Read the model definition and answer for the solid it produces. Units are mm, in the model's axes. Face numbers are marked on the shaded views. A direction names the side the tool comes from. Round coordinates to 2 decimals unless told otherwise and drop trailing zeros. Loops run counter-clockwise (first coordinate to the right, second up) from the corner with the lowest first, then second, coordinate; pieces in that order, holes last. Notation, with made-up numbers: (37, 24.25) - (75, 24.25) arc R30 cw to (75, 62.25) - close; hole circle Ø10 at (-32.5, 69). An arc over 180 degrees is marked (long way). Use one line per item in the form item = value. Start each with the question number.
```python
from build123d import *

# Parameters (mm, degrees)
SKETCH_W          = 46
SKETCH_H          = 22
PAD_DEPTH         = 20
SKETCH001_W       = 41
SKETCH001_H       = 17
POCKET_DEPTH      = 0.001
POCKET_DEPTH_BACK = 20.001
SKETCH002_R       = 3.62
POCKET001_DEPTH   = 3.5
SKETCH003_R       = 2
POCKET002_DEPTH   = 2.5
CHAMFER_SIZE      = 2.485
FILLET_R          = 1


with BuildPart() as part:
    # Sketch → Pad (new body)
    with BuildSketch(Plane.XZ):
        Rectangle(SKETCH_W, SKETCH_H)
    extrude(amount=PAD_DEPTH)

    # Sketch001 → Pocket (cut, two sides)
    with BuildSketch(Plane.XZ) as pocket_sk:
        Rectangle(SKETCH001_W, SKETCH001_H)
    extrude(amount=-POCKET_DEPTH, mode=Mode.SUBTRACT)
    extrude(pocket_sk.sketch, amount=POCKET_DEPTH_BACK, mode=Mode.SUBTRACT)

    # Sketch002 (on DatumPlane) → Pocket001 (cut)
    with BuildSketch(Plane(origin=(0, 0, 11), x_dir=(-1, 0, 0), z_dir=(0, 0, 1))):
        with Locations((-10.875, 10)):
            Circle(SKETCH002_R)
        with Locations((10.875, 10)):
            Circle(SKETCH002_R)
    extrude(amount=-POCKET001_DEPTH, mode=Mode.SUBTRACT)

    # Sketch003 (on DatumPlane) → Pocket002 (cut)
    with BuildSketch(Plane(origin=(0, 0, -8.5), x_dir=(-1, 0, 0), z_dir=(0, 0, 1))):
        with Locations((-10.875, 10)):
            Circle(SKETCH003_R)
        with Locations((10.875, 10)):
            Circle(SKETCH003_R)
    extrude(amount=-POCKET002_DEPTH, mode=Mode.SUBTRACT)

    # Chamfer
    chamfer_edges = [part.edges().sort_by_distance(p)[0] for p in [
        (-8.875, -10, -8.5),
        (12.875, -10, -8.5),
    ]]
    chamfer(chamfer_edges, length=CHAMFER_SIZE)

    # Fillet
    fillet_edges = [part.edges().sort_by_distance(p)[0] for p in [
        (-23, -20, 0),
        (0, -20, 11),
        (0, -20, -11),
        (23, -20, 0),
        (-20.5, -20, 0),
        (0, -20, 8.5),
        (20.5, -20, 0),
        (0, -20, -8.5),
        (-23, 0, 0),
        (0, 0, 11),
        (0, 0, -11),
        (23, 0, 0),
        (-20.5, 0, 0),
        (0, 0, 8.5),
        (20.5, 0, 0),
        (0, 0, -8.5),
        (23, -10, 11),
        (23, -10, -11),
        (-23, -10, -11),
        (-23, -10, 11),
        (-7.255, -10, 11),
        (14.495, -10, 11),
    ]]
    fillet(fillet_edges, radius=FILLET_R)


solid = part.part
```
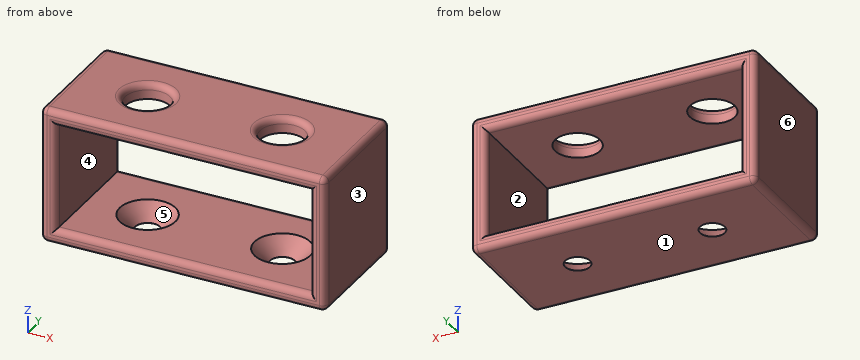
1) A cutting plane is placed at C-C on y = -4.25. Write down the section's boundary in (x, z).
2) A cutting plane is placed at D-D on y = -10. Count the separate pieces of the cut face and the enclosed holes in it, plus the area to 3 significant figures.
3) Determine the mould class of the marked faces 1, 2 and 3 for opening direction Z: +Z half, -Z half, draft (parallel to the pull), parting line (faces both ways), or undercut.
4) A cutting plane is placed at B-B on x = -1. Write down the section's boundary in (y, z).
5) A flat-ended cylindrical pin translates along its axis: pin 1 (4.5 mm diameter, centred on x = -10.875, y = -10, fed in from +Z) (3 decimals). Find the tip coordinate at first contact, or state that the pin passes through.
6) A cutting plane is placed at A-A on z = 2.75. Write down the section's boundary in (x, y).
7) For the marked faces 4, 5 and 6, determine the directions among +Z, -Z, +X, -X, +Y, -Y from which every point of the face is accessible in a straight line to the end or side of a thin tool.
8) Straight lines are drawn through the part: line 1 (X direction, y = -10, z = 8.8) (3 decimals); line 2 (Z direction, x = -8.5, y = -5.5); line 3 (X direction, y = -10.5, z = -0.75). For each, find the intervals that lie inside material, in ascending order. Write a range as from..to.
Checks:
q1.outline = (-23, -10) arc R1 ccw to (-22, -11) - (22, -11) arc R1 ccw to (23, -10) - (23, 10) arc R1 ccw to (22, 11) - (-22, 11) arc R1 ccw to (-23, 10) - close; hole (-20.5, -8.5) - (20.5, -8.5) - (20.5, 8.5) - (-20.5, 8.5) - close
q2.separate_pieces = 4
q2.enclosed_holes = 0
q2.area = 245 mm²
q3.face_1 = -Z half
q3.face_2 = undercut
q3.face_3 = draft
q4.outline = (-20, -10) arc R1 ccw to (-19, -11) - (-1, -11) arc R1 ccw to (0, -10) - (0, -9.5) arc R1 ccw to (-1, -8.5) - (-19, -8.5) arc R1 ccw to (-20, -9.5) - close; (-20, 9.5) arc R1 ccw to (-19, 8.5) - (-1, 8.5) arc R1 ccw to (0, 9.5) - (0, 10) arc R1 ccw to (-1, 11) - (-19, 11) arc R1 ccw to (-20, 10) - close
q5.pin_1 = -10.735
q6.outline = (-23, -19) arc R1 ccw to (-22, -20) - (-21.5, -20) arc R1 ccw to (-20.5, -19) - (-20.5, -1) arc R1 ccw to (-21.5, 0) - (-22, 0) arc R1 ccw to (-23, -1) - close; (20.5, -19) arc R1 ccw to (21.5, -20) - (22, -20) arc R1 ccw to (23, -19) - (23, -1) arc R1 ccw to (22, 0) - (21.5, 0) arc R1 ccw to (20.5, -1) - close
q7.face_4 = +Y, -Y
q7.face_5 = none
q7.face_6 = +Z, -Z, -X, +Y, -Y
q8.line_1 = -23..-14.495, -7.255..7.255, 14.495..23
q8.line_2 = -11..-8.5, 8.5..11
q8.line_3 = -23..-20.5, 20.5..23
